Here's the drawing with two shaded views (mm, measured from the low corner). I have some questions. A direction names the side the tool comes from. Give positions to 0.01 mm unless a question says otherwise; leave off trailing zeros. Loops run counter-clockwise (first coordinate to the right, second up) from the corner with the lowest first, then second, coordinate; pieces in that order, holes last. Notation, with made-up numbers: M -30.75,0 L 5.25,0 A33 ccw 5.25,28 Z; hole C 53,83 d8. An arc over 180 degrees is marked long. Put each result on its own line as item: value. Start each with the question number.
1) Imagine slicing it at C-C (x = 16). Write out the boundary of the cut face in (y, z).
2) For the marked faces 1 and 2, which set-ups out of +Z, -Z, +X, -X, +Y, -Y let a thin tool reach every point of the face, with its end or its side?
3) Imagine slicing it at B-B (y = 42). Write out the boundary of the cut face in (x, z).
4) Please list where these lines run through material, in increasing order: line 1 along Z through (x, y) = (25, 1.85); line 2 along Y through (x, z) = (25, 22.5); line 3 along Z through (x, y) = (47.5, 21). Write a range as from..to.
5) Imagine slicing it at A-A (z = 9.5). Write out the boundary of the cut face in (x, y), then the cut area to 3 significant figures.
6) For P1, Ø20, axis at x = 10.5, y = 34.5, coming from the -Z side; P2, Ø10, axis at x = 15, z = 7.5, coming from the +Y side; P3, Ø12, axis at x = 23.5, y = 29.5, coming from the -Z side, each with a flat end and sliding along its axis, tell me the tip position at first contact or that it passes through.
7) Imagine slicing it at D-D (z = 24). Write out the boundary of the cut face in (x, y).
8) If we mould it in two halves opening along Y, with no side actions, what happens to the marked faces 3, 4 and 5? For each: +Y half, -Y half, draft (parallel to the pull), parting line (faces both ways), or undercut.
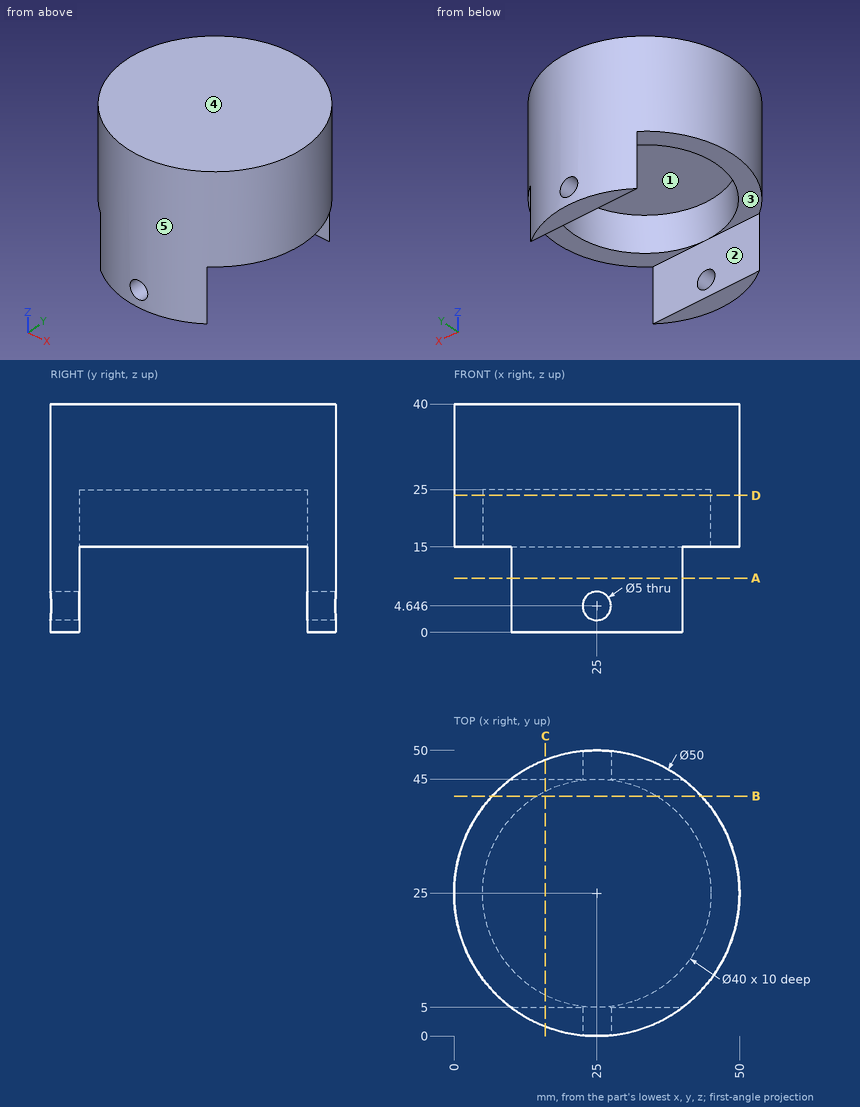
Recorded:
1. outline: M 1.68,0 L 5,0 L 5,15 L 7.14,15 L 7.14,25 L 42.86,25 L 42.86,15 L 45,15 L 45,0 L 48.32,0 L 48.32,40 L 1.68,40 Z
2. face 1: -Z
2. face 2: -Z, +X, -X
3. outline: M 6.67,15 L 14.46,15 L 14.46,25 L 35.54,25 L 35.54,15 L 43.33,15 L 43.33,40 L 6.67,40 Z
4. line 1: 0..2.15, 7.15..40
4. line 2: 0..5, 45..50
4. line 3: 15..40
5. outline: M 10,5 A25 ccw 40,5 Z; M 10,45 L 40,45 A25 ccw Z
5. area: 204 mm²
6. P1: z = 15
6. P2: y = 49.49
6. P3: z = 25
7. outline: C 25,25 d50; hole C 25,25 d40
8. face 3: undercut
8. face 4: draft
8. face 5: parting line
